Drawing for the job (mm, zero at the part's lowest x, y, z). A direction names the side the tool comes from. Give positions to 0.01 mm unless a question says otherwise; leave off trailing zeros. Order: outer loops, then holes, each group sorted by start corner. A loop starts at its lowest first (then second) coordinate and runs counter-clockwise, first axis right, second up. Notation, with made-up numbers: (33, 51) - (41, 51) arc R21 ccw to (41, 62) - close; hole circle Ø10 at (45.25, 81). An arc over 180 degrees is marked (long way). Use a Markdown table: item, result. Add a question column.
(1) Which spindle directions (+Z, -Z, +X, -X, +Y, -Y) get a long thin tool onto all of the face, cutting with end or side? Do the marked faces 1 and 2. Say none if no direction does.
(2) Wall check: line 1 (Y direction, x = 4.25, z = 7.5); line 2 (Z direction, x = 5, y = 9) (1 decimal); line 3 (X direction, y = 9.5, z = 2.75) (1 decimal). Give the ranges that are in metal, low to high.
(3) Slice it at C-C (y = 8.25). Write the cut outline in (x, z), then the cut area to 3 significant figures.
(4) Slice it at A-A (z = 7.5). Write the cut outline in (x, y), then the cut area to 3 significant figures.
(5) Slice it at B-B (x = 7.25). Write the cut outline in (y, z).
(6) Flat gauge pins, fed straight in: pin 1 (3 mm diameter, centred on y = 12, z = 5.5, fed in from +X); pin 2 (4 mm diameter, centred on x = 2, y = 1.5, fed in from +Z) (1 decimal); pin 3 (1.5 mm diameter, centred on x = 3.5, z = 6, fed in from +Y); pin 4 (2 mm diameter, centred on x = 2.5, y = 1.5, fed in from +Z) (1 decimal). Where does each tip first touch, or does it go through?
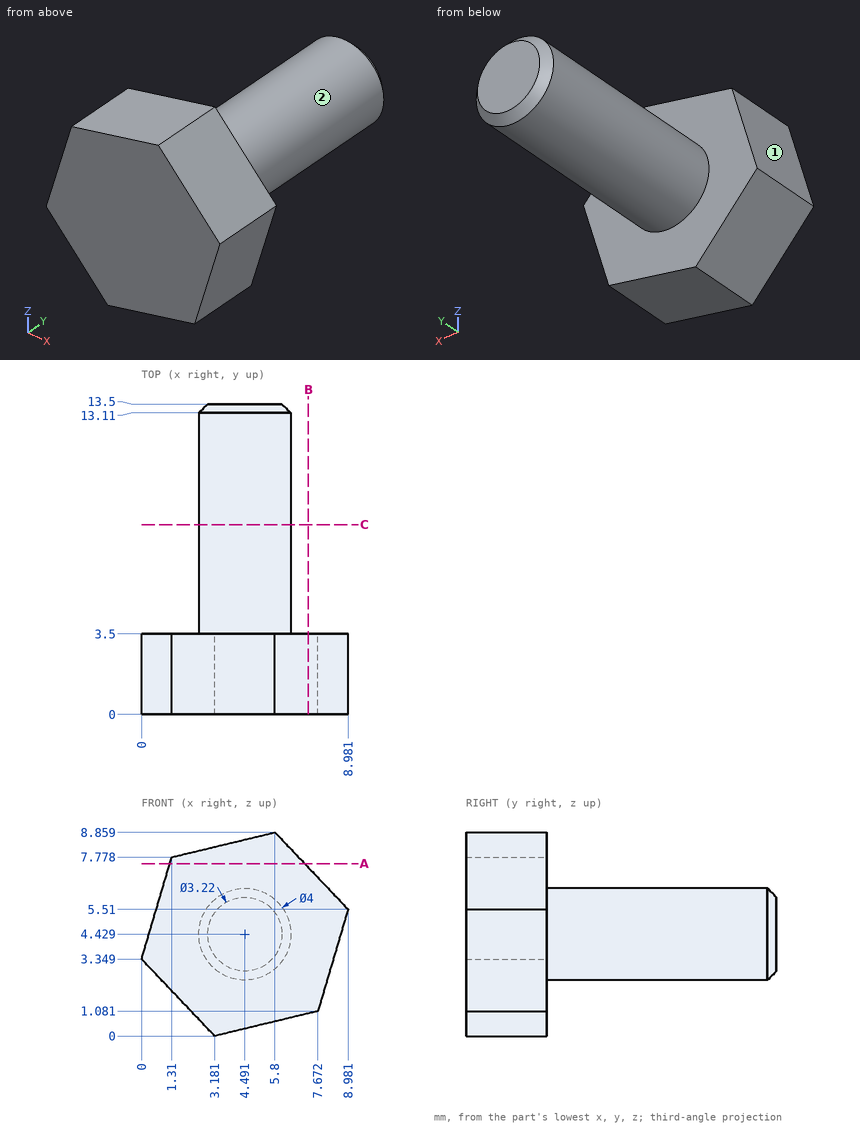
Solution:
| question | item | result |
|---|---|---|
| 1 | face 1 | +Z, -X, +Y, -Y |
| 1 | face 2 | +Y |
| 2 | line 1 | 0 to 3.5 |
| 2 | line 2 | 2.5 to 6.4 |
| 2 | line 3 | 3.4 to 5.6 |
| 3 | outline | circle Ø4 at (4.49, 4.43) |
| 3 | area | 12.6 mm2 |
| 4 | outline | (1.23, 0) - (7.09, 0) - (7.09, 3.5) - (1.23, 3.5) - close |
| 4 | area | 20.5 mm2 |
| 5 | outline | (0, 0.98) - (3.5, 0.98) - (3.5, 7.33) - (0, 7.33) - close |
| 6 | pin 1 | x = 6.49 |
| 6 | pin 2 | z = 8.4 |
| 6 | pin 3 | y = 13.5 |
| 6 | pin 4 | z = 8.3 |
